```python
from build123d import *

# Parameters (mm, degrees)
SKETCH1_W           = 96.52
SKETCH1_H           = 86.36
SKETCH1_R           = 1.27
SKETCH1_W_2         = 5.052423249
SKETCH1_H_2         = 12.313816371
SKETCH1_H_3         = 39.972542374
BOSS_EXTRUDE1_DEPTH = 1.5


with BuildPart() as part:
    # Sketch1 → Boss-Extrude1 (new body)
    with BuildSketch(Plane(origin=(0, 0, 0), x_dir=(1, 0, 0), z_dir=(0, 1, 0))):
        Rectangle(SKETCH1_W, SKETCH1_H)
        with Locations(Location((-45.421176471, 40.64, 0), (0, 0, 270))):
            Circle(SKETCH1_R, mode=Mode.SUBTRACT)
        with Locations(Location((45.421176471, 40.64, 0), (0, 0, 270))):
            Circle(SKETCH1_R, mode=Mode.SUBTRACT)
        with Locations(Location((-45.421176471, -40.64, 0), (0, 0, 270))):
            Circle(SKETCH1_R, mode=Mode.SUBTRACT)
        with Locations(Location((45.421176471, -40.64, 0), (0, 0, 270))):
            Circle(SKETCH1_R, mode=Mode.SUBTRACT)
        with Locations((-42.894964847, 26.371121385)):
            Rectangle(SKETCH1_W_2, SKETCH1_H_2, mode=Mode.SUBTRACT)
        with Locations((-42.894964847, -12.654204345)):
            Rectangle(SKETCH1_W_2, SKETCH1_H_3, mode=Mode.SUBTRACT)
    extrude(amount=BOSS_EXTRUDE1_DEPTH)


solid = part.part
```
The model under review builds one solid part; all positions refer to its coordinate system, in mm. Round coordinates to 2 decimals unless told otherwise and drop trailing zeros. Loops run counter-clockwise (first coordinate to the right, second up) from the corner with the lowest first, then second, coordinate; pieces in that order, holes last. Notation, with made-up numbers: (-40, 58) -> (-23, 58) arc R19 ccw to (-23, 67) -> close; hole circle Ø6 at (-32, -9). An arc over 180 degrees is marked (long way). Answer as a JSON object with one key per item and string values. Group by question number.
1) For pin 1 Ø4 at (x, z) = (-45.42, -40.64) entering from -Y; pin 2 Ø1.5 at (x, z) = (45.42, -40.64) entering from -Y, all flat-tipped, find the tip position at first contact; note any pin that passes through.
2) Mouldability with a two-part tool opening along X and no side actions: class faces 1 (the face through (-1, 0, -1)), 2 (the face through (-46.548, 0.74, 41.226)) as released by +X, released by -X, zero draft, split by the parting line, or undercut.
3) We need section B-B on z = 17.5. Write out the cut boundary in (x, y).
4) We need section A-A on z = -40.64. Write out the cut boundary in (x, y), then the cut area to 3 significant figures.
5) We need section C-C on y = 0.4. Write out the cut boundary in (x, z), then the cut area to 3 significant figures.
6) For line 1 (X direction, y = 1.1, z = -40.64); line 2 (Z direction, x = -42.5, y = 0.8); line 3 (X direction, y = 1.45, z = 1.5), list the stretches that pass through material, from the lowest coordinate up. Write a range as [from, to].
Result set:
{
 "1": {"pin 1": "y = 0", "pin 2": "through"},
 "2": {"face 1": "zero draft", "face 2": "undercut"},
 "3": {"outline": "(-48.26, 0) -> (-45.42, 0) -> (-45.42, 1.5) -> (-48.26, 1.5) -> close; (-40.37, 0) -> (48.26, 0) -> (48.26, 1.5) -> (-40.37, 1.5) -> close"},
 "4": {"outline": "(-48.26, 0) -> (-46.69, 0) -> (-46.69, 1.5) -> (-48.26, 1.5) -> close; (-44.15, 0) -> (44.15, 0) -> (44.15, 1.5) -> (-44.15, 1.5) -> close; (46.69, 0) -> (48.26, 0) -> (48.26, 1.5) -> (46.69, 1.5) -> close", "area": "137 mm²"},
 "5": {"outline": "(-48.26, -43.18) -> (48.26, -43.18) -> (48.26, 43.18) -> (-48.26, 43.18) -> close; hole circle Ø2.54 at (-45.42, -40.64); hole circle Ø2.54 at (-45.42, 40.64); hole (-45.42, -32.53) -> (-40.37, -32.53) -> (-40.37, -20.21) -> (-45.42, -20.21) -> close; hole (-45.42, -7.33) -> (-40.37, -7.33) -> (-40.37, 32.64) -> (-45.42, 32.64) -> close; hole circle Ø2.54 at (45.42, -40.64); hole circle Ø2.54 at (45.42, 40.64)", "area": "8,050 mm²"},
 "6": {"line 1": "[-48.26, -46.69], [-44.15, 44.15], [46.69, 48.26]", "line 2": "[-43.18, -32.53], [-20.21, -7.33], [32.64, 43.18]", "line 3": "[-48.26, -45.42], [-40.37, 48.26]"}
}
